Input: dimensioned drawing with shaded views. Units: mm. Origin: part minimum x, y, z. Round coordinates to 2 decimals unless told otherwise and drop trailing zeros. Loops run counter-clockwise (first coordinate to the right, second up) from the corner with the lowest first, then second, coordinate; pieces in that order, holes last. Notation, with made-up numbers: (-13.75, 39) - (43.25, 39) arc R13 cw to (43.25, 59) - close; hole circle Ø6 at (71, 1). An arc over 180 degrees is marked (long way). One line per question, with ' | ' between items. Start each with the question number.
1. Pin query (flat end, axial travel): pin 1 (1.8 mm diameter, centred on x = 3.5, z = 135.5, fed in from +Y); pin 2 (3 mm diameter, centred on x = 1, y = 41, fed in from -Z); pin 3 (3 mm diameter, centred on x = 4.5, y = 35.5, fed in from +Z). Return the tip coordinate at first contact, or that it passes through.
2. Cut plane B-B (x = 3.9). Return loops of the section in (y, z).
3. Cut plane A-A (y = 42). Return loops of the section in (x, z), then the cut area to 3 significant figures.
4. Ray query, line 1 (Z direction, x = 4.75, y = 27); line 2 (Y direction, x = 5.25, z = 7.5). Return the intervals inside material, ascending.
5. Cut plane C-C (z = 27). Return loops of the section in (x, y), then the cut area to 3 significant figures.
6. Cut plane D-D (y = 34). Return loops of the section in (x, z), then the cut area to 3 significant figures.
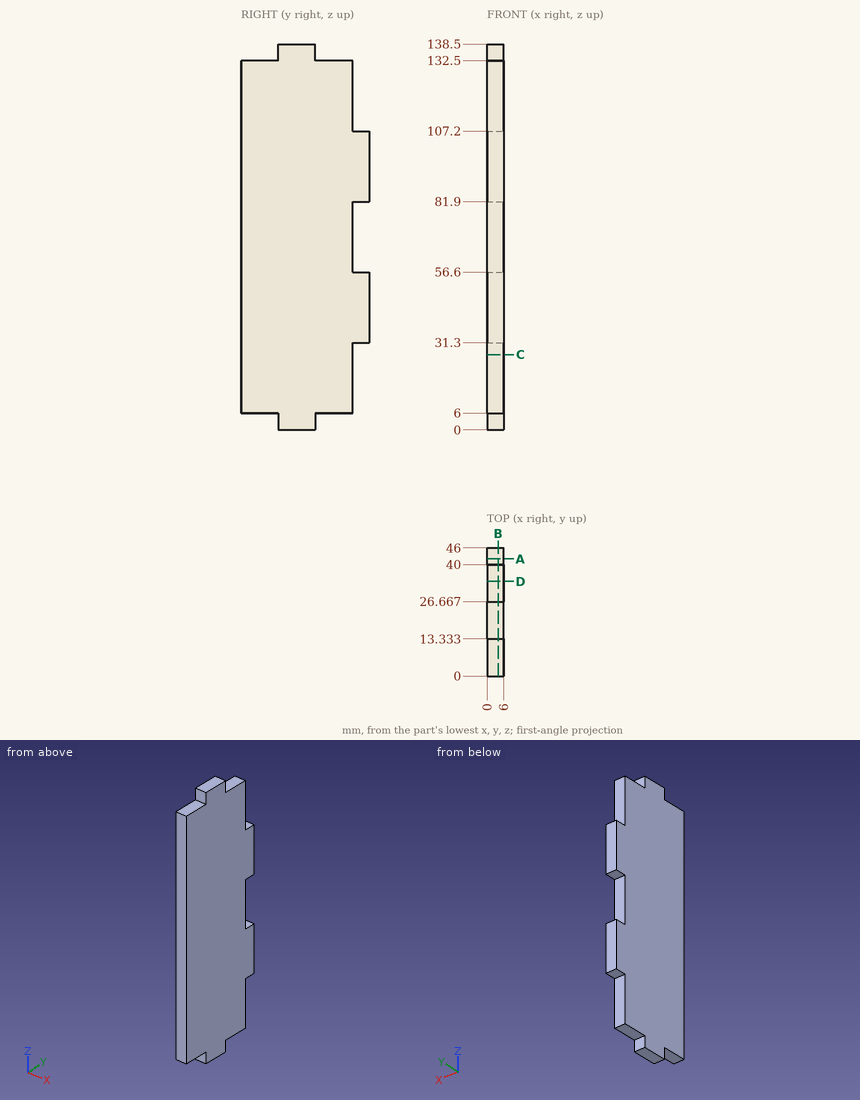
Answers follow:
1) pin 1: stops at y = 26.67 | pin 2: stops at z = 6 | pin 3: stops at z = 132.5
2) outline: (0, 6) - (13.33, 6) - (13.33, 0) - (26.67, 0) - (26.67, 6) - (40, 6) - (40, 31.3) - (46, 31.3) - (46, 56.6) - (40, 56.6) - (40, 81.9) - (46, 81.9) - (46, 107.2) - (40, 107.2) - (40, 132.5) - (26.67, 132.5) - (26.67, 138.5) - (13.33, 138.5) - (13.33, 132.5) - (0, 132.5) - close
3) outline: (0, 31.3) - (6, 31.3) - (6, 56.6) - (0, 56.6) - close; (0, 81.9) - (6, 81.9) - (6, 107.2) - (0, 107.2) - close | area: 304 mm2
4) line 1: z = 6 to 132.5 | line 2: y = 0 to 40
5) outline: (0, 0) - (6, 0) - (6, 40) - (0, 40) - close | area: 240 mm2
6) outline: (0, 6) - (6, 6) - (6, 132.5) - (0, 132.5) - close | area: 759 mm2
